For this review, use the dimensioned drawing (mm, ordinates from the lowest corner) and the shaded views. A direction names the side the tool comes from. Coordinates: 2 decimals unless noted, no trailing zeros. Order: outer loops, then holes, each group sorted by start corner. A loop starts at its lowest first (then second) coordinate and runs counter-clockwise, first axis right, second up. Notation, with made-up numbers: (-10, -9.5) -> (23, -9.5) arc R25 cw to (23, 27.5) -> close; hole circle Ø7 at (79, 27.5). An arc over 180 degrees is marked (long way). Return JSON: item names as keys, results as strings. Group by question number.
Item 1: For line 1 along Z through (x, y) = (15, 4.4); line 2 along X through (y, z) = (0.7, 19.25) (1 decimal); line 3 along Z through (x, y) = (8, 3.1), list the stretches that pass through material, from the lowest coordinate up.
Item 2: Take a section at C-C (x = 17.5). Write out the cut boundary in (y, z).
Item 3: Draft analysis for pull direction X (two halves, no side actions). For the marked faces 1, 2, 3 and 4, state which applies: +X half, -X half, draft (parallel to the pull), parting line (faces both ways), or undercut.
Item 4: Take a section at D-D (z = 10.5). Write out the cut boundary in (x, y).
Item 5: Machinability: for the marked faces 5 and 6, which of the approach directions +Z, -Z, +X, -X, +Y, -Y give a long, thin tool a straight path to every point of the face, cutting with its end or side? Answer none if there is none.
Item 6: Insertion check: pin 1 (2 mm diameter, centred on y = 1.5, z = 8.5, fed in from +X) (1 decimal); pin 2 (1.5 mm diameter, centred on x = 14, z = 16, fed in from -Y); pin 3 (4.5 mm diameter, centred on x = 16, z = 15.5, fed in from -Y); pin 4 (1 mm diameter, centred on x = 12, y = 1, fed in from -Z). Each pin has a flat end and moves straight along its axis. Give the tip position at first contact, or say it passes through.
Item 7: Take a section at A-A (y = 0.65). Write out the cut boundary in (x, z).
Item 8: Take a section at B-B (z = 15). Write out the cut boundary in (x, y), then the cut area to 3 significant figures.
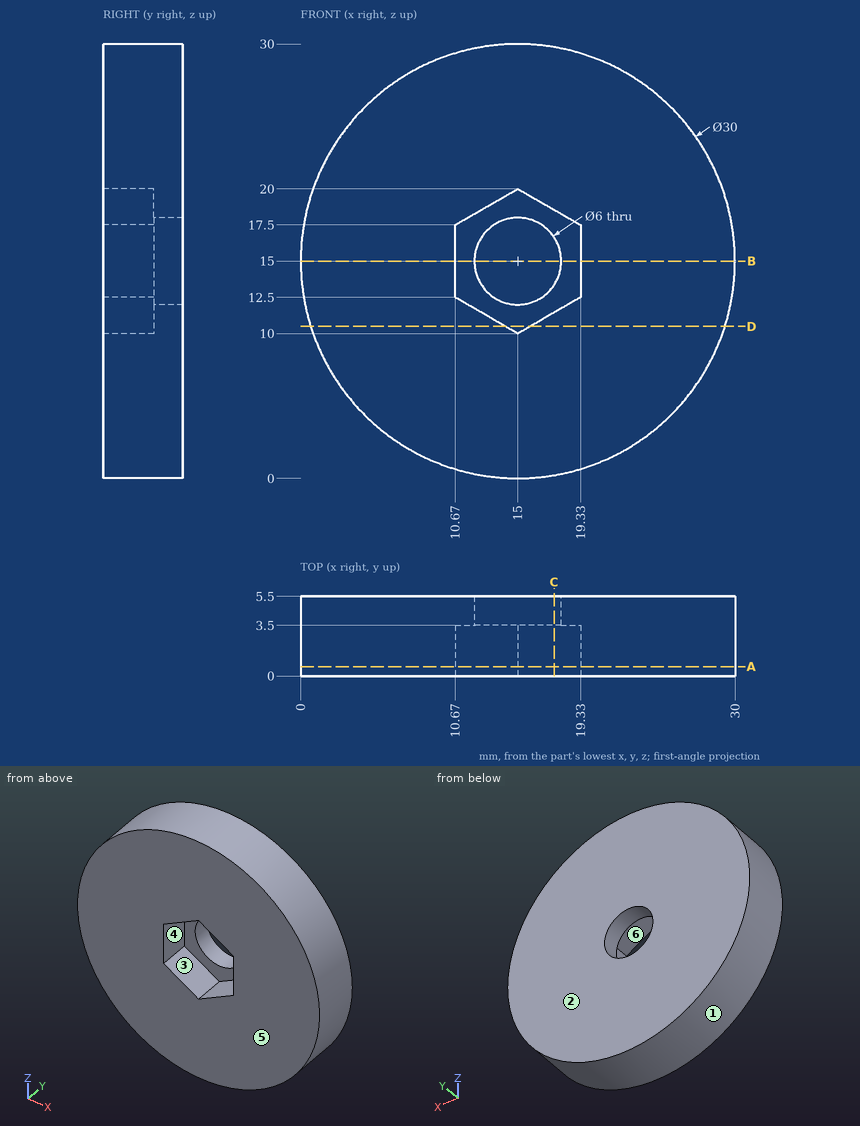
Findings below:
{
 "1": {"line 1": "z = 0 to 12, 18 to 30", "line 2": "x = 0.6 to 13.7, 16.3 to 29.4", "line 3": "z = 1.73 to 28.27"},
 "2": {"outline": "(0, 0.21) -> (5.5, 0.21) -> (5.5, 13.34) -> (3.5, 13.34) -> (3.5, 11.44) -> (0, 11.44) -> close; (0, 18.56) -> (3.5, 18.56) -> (3.5, 16.66) -> (5.5, 16.66) -> (5.5, 29.79) -> (0, 29.79) -> close"},
 "3": {"face 1": "parting line", "face 2": "draft", "face 3": "undercut", "face 4": "undercut"},
 "4": {"outline": "(0.69, 0) -> (14.13, 0) -> (14.13, 3.5) -> (15.87, 3.5) -> (15.87, 0) -> (29.31, 0) -> (29.31, 5.5) -> (0.69, 5.5) -> close"},
 "5": {"face 5": "+Z, -Z, +X, -X, -Y", "face 6": "-Y"},
 "6": {"pin 1": "stops at x = 29", "pin 2": "passes through", "pin 3": "stops at y = 3.5", "pin 4": "stops at z = 0.21"},
 "7": {"outline": "circle Ø30 at (15, 15); hole (10.67, 12.5) -> (15, 10) -> (19.33, 12.5) -> (19.33, 17.5) -> (15, 20) -> (10.67, 17.5) -> close"},
 "8": {"outline": "(0, 0) -> (10.67, 0) -> (10.67, 3.5) -> (12, 3.5) -> (12, 5.5) -> (0, 5.5) -> close; (18, 3.5) -> (19.33, 3.5) -> (19.33, 0) -> (30, 0) -> (30, 5.5) -> (18, 5.5) -> close", "area": "123 mm2"}
}
